Design review of the part built by this model. Coordinates are the model's own, in mm. A direction names the side the tool comes from. Round coordinates to 2 decimals unless told otherwise and drop trailing zeros. Order: outer loops, then holes, each group sorted by start corner. A loop starts at its lowest first (then second) coordinate and runs counter-clockwise, first axis right, second up. Notation, with made-up numbers: (72.5, 66.5) - (93.5, 66.5) arc R11 ccw to (93.5, 80.5) - close; hole circle Ø5 at (-35, -6.75). An arc over 180 degrees is marked (long way). Answer as a JSON object with one key per item and string values. Group by question number.
from build123d import *

# Parameters (mm, degrees)
BOSS_EXTRU_1_DEPTH      = 18
BOSS_EXTRU_1_DEPTH_BACK = 18
CONG_1_R                = 10
ESQUISSE2_W             = 12.5
ESQUISSE2_H             = 17
ENL_V_MAT_EXTRU_1_DEPTH = 3


with BuildPart() as part:
    # Esquisse1 → Boss.-Extru.1 (new, two sides: drawn at the far end of the back side and taken through both)
    with BuildSketch(Plane.XY.offset(-BOSS_EXTRU_1_DEPTH_BACK)):
        Polygon((0, 0), (0, 80), (13.680805733, 117.587704831), (16.499883595, 116.561644401), (3.192533317, 80), (3.192533317, 0), align=None)
    extrude(amount=BOSS_EXTRU_1_DEPTH + BOSS_EXTRU_1_DEPTH_BACK)

    # Congé1
    cong_1_edges = [part.edges().sort_by_distance(p)[0] for p in [
        (0, 80, 0),
    ]]
    fillet(cong_1_edges, radius=CONG_1_R)

    # Esquisse2 → Enlèv. mat.-Extru.1 (cut)
    with BuildSketch(Plane(origin=(-25.711504387, 9.358222275, 0), x_dir=(0, 0, 1), z_dir=(-0.9396926207859093, 0.34202014332566644, 0))):
        with Locations((0, 106.675409663)):
            Rectangle(ESQUISSE2_W, ESQUISSE2_H)
    extrude(amount=-ENL_V_MAT_EXTRU_1_DEPTH, mode=Mode.SUBTRACT)


solid = part.part
1. Clearance check with flat-ended pins moving along their axes: P1, Ø1.5, axis at y = 82.5, z = -4.5, coming from the +X side; P2, Ø2, axis at y = 22, z = 5.5, coming from the +X side; P3, Ø6, axis at x = 11, z = 10.5, coming from the +Y side. State where each tip first meets the part, or that it passes through.
2. Take a section at D-D, the plane y = 98. Give the boundary of the cut face in (x, z), then the cut area to 3 significant figures.
3. Take a section at B-B, the plane x = 15.25. Give the boundary of the cut face in (y, z).
4. Mouldability with a two-part tool opening along Z and no side actions: class faces 4 (the flat face through (3, 59, 18)), 5 (the flat face through (2, 0, 0)), 6 (the flat face through (12, 109, -6.25)), 7 (the flat face through (3, 59, -18)) as pulls with the +Z half, pulls with the -Z half, needs draft (parallel to the pull), parting line crosses it, or undercut.
5. To check wall thickness, follow line 1 (X direction, y = 62, z = -13); line 2 (X direction, y = 85.5, z = 9.5). State the ranges of each line that lie inside material, in increasing order. Write a range as from..to.
6. Tool access review of faces 1 (the flat face through (9.256, 101.107, -0.087)), 2 (the flat face through (3.193, 41, 0)), 3 (the flat face through (15.07, 117.08, -12.21)): name each direction out of +Z, -Z, +X, -X, +Y, -Y from which nothing blocks a thin tool from reaching the whole face with its end or side.
7. Take a section at C-C, the plane z = -2.5. Give the boundary of the cut face in (x, y), then the cut area to 3 significant figures.
8. Take a section at A-A, the plane z = 11. Give the boundary of the cut face in (x, y), then the cut area to 3 significant figures.
Response values:
{
 "1": {"P1": "x = 4.38", "P2": "x = 3.19", "P3": "y = 117.59"},
 "2": {"outline": "(6.55, -18) - (9.74, -18) - (9.74, 18) - (6.55, 18) - close", "area": "115 mm2"},
 "3": {"outline": "(113.13, -18) - (117.02, -18) - (117.02, -6.25) - (113.13, -6.25) - close; (113.13, 6.25) - (117.02, 6.25) - (117.02, 18) - (113.13, 18) - close"},
 "4": {"face 4": "pulls with the +Z half", "face 5": "needs draft", "face 6": "undercut", "face 7": "pulls with the -Z half"},
 "5": {"line 1": "0..3.19", "line 2": "2..5.19"},
 "6": {"face 1": "+X, +Y", "face 2": "+Z, -Z, +X, -Y", "face 3": "+Z, -Z, +X, +Y"},
 "7": {"outline": "(0, 0) - (3.19, 0) - (3.19, 80) - (10.69, 100.59) - (7.87, 101.61) - (0.6, 81.66) arc R10 ccw to (0, 78.24) - close", "area": "323 mm2"},
 "8": {"outline": "(0, 0) - (3.19, 0) - (3.19, 80) - (16.5, 116.56) - (13.68, 117.59) - (0.6, 81.66) arc R10 ccw to (0, 78.24) - close", "area": "374 mm2"}
}
